Autodesk Inventor part; units mm, degrees
ref_plane "YZ Plane" through (0, 0, 0) normal (1, 0, 0) x (0, 1, 0)
ref_plane "XZ Plane" through (0, 0, 0) normal (0, 1, 0) x (-1, 0, 0)
ref_plane "XY Plane" through (0, 0, 0) normal (0, 0, 1) x (1, 0, 0)
sketch "Sketch1" plane through (0, 0, 0) normal (0, 1, 0) x (-1, 0, 0)
  arc A0 (210.5939, -215.9) -> (210.5939, 215.9) centre (0, 0) ccw
  line L0 (470.9439, 215.9) -> (470.9439, -215.9)
  line L1 (470.9439, 215.9) -> (407.4439, 215.9)
  line L2 (407.4439, 215.9) -> (407.4439, 95.25)
  line L3 (407.4439, 95.25) -> (331.2439, 95.25)
  line L4 (331.2439, 95.25) -> (331.2439, 215.9)
  line L5 (470.9439, -215.9) -> (407.4439, -215.9)
  line L6 (407.4439, -215.9) -> (407.4439, -95.25)
  line L7 (407.4439, -95.25) -> (331.2439, -95.25)
  line L8 (331.2439, -95.25) -> (331.2439, -215.9)
  line L9 (331.2439, 215.9) -> (210.5939, 215.9)
  line L10 (331.2439, -215.9) -> (210.5939, -215.9)
  circle A1 centre (458.2439, 203.2) radius 2.4892
  circle A2 centre (445.5439, 203.2) radius 2.4892
  circle A3 centre (432.8439, 203.2) radius 2.4892
  circle A4 centre (420.1439, 203.2) radius 2.4892
  circle A5 centre (318.5439, 203.2) radius 2.4892
  circle A6 centre (305.8439, 203.2) radius 2.4892
  circle A7 centre (293.1439, 203.2) radius 2.4892
  circle A8 centre (280.4439, 203.2) radius 2.4892
  circle A9 centre (267.7439, 203.2) radius 2.4892
  circle A10 centre (255.0439, 203.2) radius 2.4892
  circle A11 centre (242.3439, 203.2) radius 2.4892
  circle A12 centre (229.6439, 203.2) radius 2.4892
  line L11 (597.6164, 0) -> (168.2721, 0) construction
  circle A13 centre (458.2439, -203.2) radius 2.4892
  circle A14 centre (445.5439, -203.2) radius 2.4892
  circle A15 centre (432.8439, -203.2) radius 2.4892
  circle A16 centre (420.1439, -203.2) radius 2.4892
  circle A17 centre (318.5439, -203.2) radius 2.4892
  circle A18 centre (305.8439, -203.2) radius 2.4892
  circle A19 centre (293.1439, -203.2) radius 2.4892
  circle A20 centre (280.4439, -203.2) radius 2.4892
  circle A21 centre (267.7439, -203.2) radius 2.4892
  circle A22 centre (255.0439, -203.2) radius 2.4892
  circle A23 centre (242.3439, -203.2) radius 2.4892
  circle A24 centre (229.6439, -203.2) radius 2.4892
  dimension "d0" = 603.2002
  dimension "d1" = 431.8
  dimension "d2" = 63.5
  dimension "d3" = 120.65
  dimension "d4" = 76.2
  dimension "d5" = 63.5
  dimension "d6" = 120.65
  dimension "d7" = 76.2
  dimension "d8" = 120.65
  dimension "d9" = 120.65
  dimension "d10" = 4.9784
  dimension "d11" = 12.7
  dimension "d12" = 12.7
  dimension "d15" = 12.7
  dimension "d20" = 4.9784
  dimension "d21" = 12.7
  dimension "d22" = 12.7
  dimension "d25" = 12.7
  dimension "d30" = 12.7
extrude "Extrusion1" add sketch "Sketch1" along normal blind 6.35
sketch "Sketch2" plane through (0, 6.35, 0) normal (0, 1, 0) x (1, 0, 0)
  line L0 (-407.4439, -215.9) -> (-407.4439, -95.25)
  line L1 (-407.4439, -95.25) -> (-331.2439, -95.25)
  line L2 (-331.2439, -95.25) -> (-331.2439, -215.9)
  line L3 (-331.2439, -215.9) -> (-210.5939, -215.9)
  arc A0 (-210.5939, 215.9) -> (-210.5939, -215.9) centre (0, 0) ccw
  line L4 (-210.5939, 215.9) -> (-331.2439, 215.9)
  line L5 (-331.2439, 215.9) -> (-331.2439, 95.25)
  line L6 (-331.2439, 95.25) -> (-407.4439, 95.25)
  line L7 (-407.4439, 95.25) -> (-407.4439, 215.9)
  line L8 (-407.4439, 215.9) -> (-470.9439, 215.9)
  line L9 (-470.9439, 215.9) -> (-470.9439, -215.9)
  line L10 (-470.9439, -215.9) -> (-407.4439, -215.9)
  circle A1 centre (-305.8439, 203.2) radius 2.4892
  circle A2 centre (-458.2439, 203.2) radius 2.4892
  circle A3 centre (-432.8439, 203.2) radius 2.4892
  circle A4 centre (-420.1439, 203.2) radius 2.4892
  circle A5 centre (-305.8439, -203.2) radius 2.4892
  circle A6 centre (-318.5439, -203.2) radius 2.4892
  circle A7 centre (-420.1439, -203.2) radius 2.4892
  circle A8 centre (-432.8439, -203.2) radius 2.4892
  circle A9 centre (-445.5439, -203.2) radius 2.4892
  circle A10 centre (-458.2439, -203.2) radius 2.4892
  circle A11 centre (-445.5439, 203.2) radius 2.4892
  circle A12 centre (-318.5439, 203.2) radius 2.4892
  circle A13 centre (-293.1439, 203.2) radius 2.4892
  circle A14 centre (-280.4439, 203.2) radius 2.4892
  circle A15 centre (-267.7439, 203.2) radius 2.4892
  circle A16 centre (-255.0439, 203.2) radius 2.4892
  circle A17 centre (-242.3439, 203.2) radius 2.4892
  circle A18 centre (-229.6439, 203.2) radius 2.4892
  circle A19 centre (-229.6439, -203.2) radius 2.4892
  circle A20 centre (-242.3439, -203.2) radius 2.4892
  circle A21 centre (-255.0439, -203.2) radius 2.4892
  circle A22 centre (-267.7439, -203.2) radius 2.4892
  circle A23 centre (-280.4439, -203.2) radius 2.4892
  circle A24 centre (-293.1439, -203.2) radius 2.4892
extrude "Extrusion2" cut sketch "Sketch2" against normal blind 3.175
properties part number "Polycarbonate-Note-Intakaur-Cover" material "Polycarbonate, Smoke"
Work out the finished part from the listing and answer in its coordinate system (mm). Give positions to 0.01 mm unless a question says otherwise; leave off trailing zeros. Loops run counter-clockwise (first coordinate to the right, second up) from the corner with the lowest first, then second, coordinate; pieces in that order, holes last. Notation, with made-up numbers: (23.25, -18) - (71.25, -18) arc R23 ccw to (71.25, 1) - close; hole circle Ø6 at (53.5, 81.5). An arc over 180 degrees is marked (long way). Answer in a Markdown table with one row per item. Add a question column.
Q1. Each of these flat-tipped pins is pushed along its axis until it touches: P1, Ø1, axis at x = -360.5, y = 1, coming from the +Z side; P2, Ø4, axis at x = -318.54, z = -203.2, coming from the +Y side; P3, Ø1, axis at y = 1, z = 155, coming from the +X side; P4, Ø1, axis at y = 1.5, z = 129, coming from the +X side. Where does it stop, or does it pass through?
Q2. The part is cut by section B-B (x = -348.5). Determine the outline of the cut face in (y, z) (3 decimals), and give its area (3 significant figures).
Q3. The part is cut by section A-A (y = 2.3). State how many separate pieces and enclosed holes the cut face has, and give its area (3 significant figures).
Q4. Consider line 1 along Z through (x, y) = (-432, 0.9); line 2 along Z through (x, y) = (-227.5, 0.25); line 3 along Z through (x, y) = (-266, 2.05). Determine where each line is inside the solid, lowest interval first.
Q5. The part is cut by section C-C (z = -77). Determine the outline of the cut face in (x, y) (3 decimals), and give its area (3 significant figures).
Solution:
| question | item | result |
|---|---|---|
| 1 | P1 | stops at z = 95.25 |
| 1 | P2 | passes through |
| 1 | P3 | stops at x = -258.42 |
| 1 | P4 | stops at x = -272.38 |
| 2 | outline | (0, -95.25) - (3.175, -95.25) - (3.175, 95.25) - (0, 95.25) - close |
| 2 | area | 605 mm² |
| 3 | separate pieces | 1 |
| 3 | enclosed holes | 24 |
| 3 | area | 66,500 mm² |
| 4 | line 1 | z = -215.9 to -205.54, -200.86 to 200.86, 205.54 to 215.9 |
| 4 | line 2 | z = -215.9 to -204.46, -201.94 to -198.01, 198.01 to 201.94, 204.46 to 215.9 |
| 4 | line 3 | z = -215.9 to -204.98, -201.42 to -142.15, 142.15 to 201.42, 204.98 to 215.9 |
| 5 | outline | (-470.944, 0) - (-291.605, 0) - (-291.605, 3.175) - (-470.944, 3.175) - close |
| 5 | area | 569 mm² |
